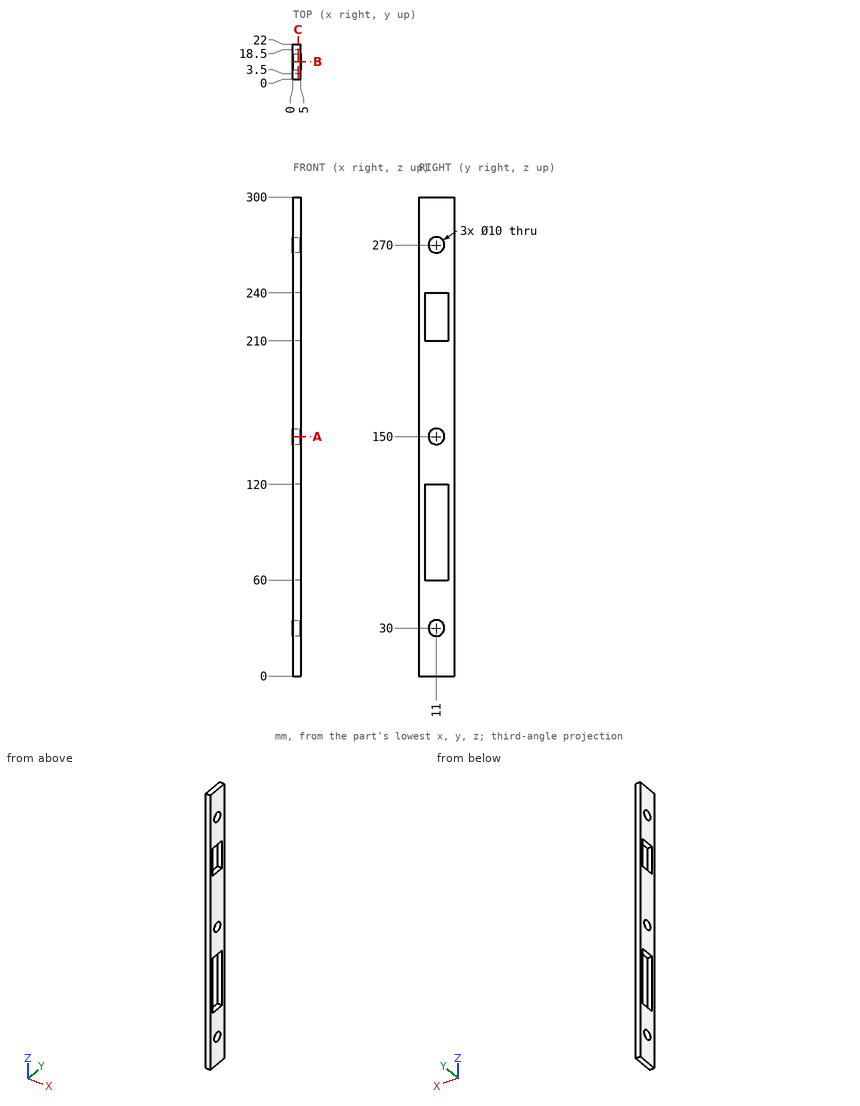
Drawing for the job (mm, zero at the part's lowest x, y, z). Round coordinates to 2 decimals unless told otherwise and drop trailing zeros. Loops run counter-clockwise (first coordinate to the right, second up) from the corner with the lowest first, then second, coordinate; pieces in that order, holes last. Notation, with made-up numbers: (25, 72) -> (56, 72) arc R19 cw to (56, 101) -> close; hole circle Ø9 at (-7, -29). An arc over 180 degrees is marked (long way). Answer in a Markdown table with one row per item.
Item 1: Pin check, flat tips, straight feed: pin 1 (4 mm diameter, centred on y = 7, z = 185, fed in from -X); pin 2 (9 mm diameter, centred on y = 11, z = 270, fed in from -X). Stop position of each tip, or through.
Answers below:
| item | result |
|---|---|
| pin 1 | stops at x = 0 |
| pin 2 | passes through |
Item 2: Saw through at B-B (y = 11). Write the cut outline in (x, z).
Answers below:
| item | result |
|---|---|
| outline | (0, 0) -> (5, 0) -> (5, 25) -> (0, 25) -> close; (0, 35) -> (5, 35) -> (5, 60) -> (0, 60) -> close; (0, 120) -> (5, 120) -> (5, 145) -> (0, 145) -> close; (0, 155) -> (5, 155) -> (5, 210) -> (0, 210) -> close; (0, 240) -> (5, 240) -> (5, 265) -> (0, 265) -> close; (0, 275) -> (5, 275) -> (5, 300) -> (0, 300) -> close |
Item 3: Saw through at C-C (x = 3.2). Write the cut outline in (y, z), and give its area (3 significant figures).
Answers below:
| item | result |
|---|---|
| outline | (0, 0) -> (22, 0) -> (22, 300) -> (0, 300) -> close; hole (3.5, 60) -> (18.5, 60) -> (18.5, 120) -> (3.5, 120) -> close; hole (3.5, 210) -> (18.5, 210) -> (18.5, 240) -> (3.5, 240) -> close; hole circle Ø10 at (11, 30); hole circle Ø10 at (11, 150); hole circle Ø10 at (11, 270) |
| area | 5,010 mm² |
Item 4: Drill centre lines: L1, parallel to Y at x = 2.85, z = 150; L2, parallel to Y at x = 2.6, z = 216.5; L3, parallel to Z at x = 3.75, y = 10.5. Where is each one in solid material? Low to high. Write a range as [from, to].
Answers below:
| item | result |
|---|---|
| L1 | y = [0, 6], [16, 22] |
| L2 | y = [0, 3.5], [18.5, 22] |
| L3 | z = [0, 25.03], [34.97, 60], [120, 145.03], [154.97, 210], [240, 265.03], [274.97, 300] |
Item 5: Saw through at A-A (z = 150). Write the cut outline in (x, y), and give its area (3 significant figures).
Answers below:
| item | result |
|---|---|
| outline | (0, 0) -> (5, 0) -> (5, 6) -> (0, 6) -> close; (0, 16) -> (5, 16) -> (5, 22) -> (0, 22) -> close |
| area | 60.0 mm² |
